from build123d import *

# Parameters (mm, degrees)
EXTRUDE_1_DEPTH     = 15
SKETCH_5_R          = 15
EXTRUDE_3_DEPTH     = 17
SKETCH_9_R          = 10.1
CUT_EXTRUDE_2_DEPTH = 2


with BuildPart() as part:
    # ｽｹｯﾁ4 → ﾎﾞｽ - 押し出し1 (new body)
    with BuildSketch(Plane.XY):
        with BuildLine():
            ThreePointArc((14.933936552, -1.40625), (0, 15), (-14.933936552, -1.40625))
            ThreePointArc((-14.933936552, -1.40625), (0, -160), (14.933936552, -1.40625))
        make_face()
    extrude(amount=EXTRUDE_1_DEPTH)

    # ｽｹｯﾁ5 → ﾎﾞｽ - 押し出し3 (add)
    with BuildSketch(Plane.XY.offset(15)):
        with Locations(Location((0, 0, 0), (0, 0, 185.379378991))):
            Circle(SKETCH_5_R)
    extrude(amount=EXTRUDE_3_DEPTH)

    # ｽｹｯﾁ9 → ｶｯﾄ - 押し出し2 (cut)
    with BuildSketch(Plane.XY.offset(32)):
        Circle(SKETCH_9_R)
    extrude(amount=-CUT_EXTRUDE_2_DEPTH, mode=Mode.SUBTRACT)


solid = part.part
Design review of the part built by this model. Coordinates are the model's own, in mm. Round coordinates to 2 decimals unless told otherwise and drop trailing zeros. Write each loop counter-clockwise with the first axis right and the second up, starting at its lowest first coordinate (ties: lowest second). Pieces come first, ordered by that corner, then holes. Notation, with made-up numbers: M 89.25,20.5 L 138.25,20.5 A8 cw 138.25,33.5 Z; hole C 63,38.5 d10. An arc over 180 degrees is marked long. One line per item, written item: value. Start each with the question number.
1. Take a section at A-A on x = 0. State the section outline as (y, z) points.
2. Take a section at C-C on z = 4. State the section outline as (x, y) points.
3. Clearance check with flat-ended pins moving along their axes: P1, Ø3, axis at y = -19, z = 5.5, coming from the +X side; P2, Ø1, axis at x = 15, y = -82, coming from the +Z side; P3, Ø8, axis at y = -40.5, z = 12.5, coming from the -X side; P4, Ø2, axis at x = 39.5, y = -89, coming from the -Z side. State where each tip first meets the part, or that it passes through.
4. Take a section at D-D on y = -20. State the section outline as (x, z) points.
5. Draft analysis for pull direction Y (two halves, no side actions). For faces 1 (the face through (-1, -80, 15)), 2 (the face through (0, 0, 30)), 3 (the face through (9.634, 3.034, 31.014)), 4 (the face through (-3.31, -159.93, 7.4)), state which applies: pulls with the +Y half, pulls with the -Y half, needs draft (parallel to the pull), parting line crosses it, or undercut.
6. To check wall thickness, follow probe 1 along Y at (x, z) = (0, 31); probe 2 along Z at (x, y) = (61.5, -131); probe 3 along Y at (x, z) = (1.5, 14). State the ranges of each line that lie inside material, in increasing order. Write a range as from..to.
7. Take a section at B-B on y = -80. State the section outline as (x, z) points, then the cut area to 3 significant figures.
Computed:
1. outline: M -160,0 L 15,0 L 15,32 L 10.1,32 L 10.1,30 L -10.1,30 L -10.1,32 L -15,32 L -15,15 L -160,15 Z
2. outline: M -14.93,-1.41 A80 ccw long 14.93,-1.41 A15 ccw long Z
3. P1: stops at x = 53.48
3. P2: stops at z = 15
3. P3: stops at x = -71.69
3. P4: stops at z = 0
4. outline: M -52.92,0 L 52.92,0 L 52.92,15 L -52.92,15 Z
5. face 1: needs draft
5. face 2: undercut
5. face 3: undercut
5. face 4: parting line crosses it
6. probe 1: y = -15..-10.1, 10.1..15
6. probe 2: z = 0..15
6. probe 3: y = -159.99..14.92
7. outline: M -80,0 L 80,0 L 80,15 L -80,15 Z
7. area: 2,400 mm²
